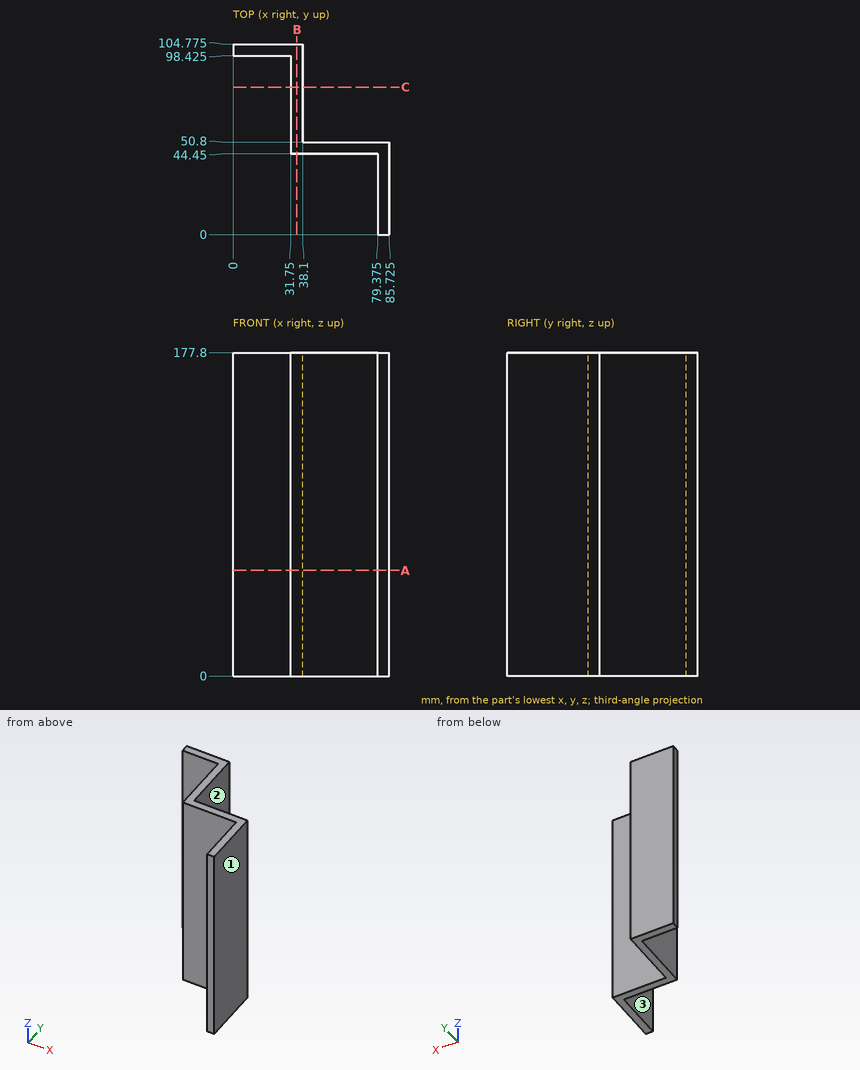
The figure shows three views and two pictorial views of one solid part (mm, origin at its lowest corner). Answer the questions. A direction names the side the tool comes from. Coordinates: 2 decimals unless noted, no trailing zeros. Write each loop counter-clockwise with the first axis right and the second up, starting at its lowest first coordinate (ties: lowest second). Pieces come first, ordered by that corner, then holes. Notation, with made-up numbers: (17, -30) -> (51, -30) arc R29 ccw to (51, 2) -> close; hole circle Ø11 at (-10.5, 24.25). An arc over 180 degrees is marked (long way). Return JSON: item names as keys, results as strings.
(1) The part is cut by section C-C on y = 81. Give the vertices of the cut face in (x, z).
Answers below:
{"outline": "(31.75, 0) -> (38.1, 0) -> (38.1, 177.8) -> (31.75, 177.8) -> close"}
(2) Which of the six approach directions +Z, -Z, +X, -X, +Y, -Y give full straight-line access (tool end or side, diameter ignored) to the marked faces 1, 2 and 3?
Answers below:
{"face 1": "+Z, -Z, +X, +Y, -Y", "face 2": "+Z, -Z, +X, +Y", "face 3": "+Z, -Z, -X, -Y"}
(3) Each of these flat-tipped pins is pushed along its axis until it touches: P1, Ø14.5, axis at x = 61, z = 105.5, coming from the +Y side; P2, Ø6, axis at x = 24.5, z = 120.5, coming from the -Y side (3 decimals); P3, Ø6, axis at x = 41.5, z = 58, coming from the -Y side; P4, Ø6, axis at x = 47, y = 55, coming from the +Z side. Where does it stop, or does it pass through?
Answers below:
{"P1": "y = 50.8", "P2": "y = 98.425", "P3": "y = 44.45", "P4": "through"}
(4) The part is cut by section B-B on x = 35. Give the vertices of the cut face in (y, z) (3 decimals).
Answers below:
{"outline": "(44.45, 0) -> (104.775, 0) -> (104.775, 177.8) -> (44.45, 177.8) -> close"}
(5) Consider line 1 along X through (y, z) = (35, 126.5) (3 decimals); line 2 along X through (y, z) = (51, 11); line 3 along Y through (x, z) = (70, 55.5). Determine where each line is inside the solid, lowest interval first. Write a range as from..to.
Answers below:
{"line 1": "79.375..85.725", "line 2": "31.75..38.1", "line 3": "44.45..50.8"}
(6) The part is cut by section A-A on z = 58. Give the vertices of the cut face in (x, y) (3 decimals).
Answers below:
{"outline": "(0, 98.425) -> (31.75, 98.425) -> (31.75, 44.45) -> (79.375, 44.45) -> (79.375, 0) -> (85.725, 0) -> (85.725, 50.8) -> (38.1, 50.8) -> (38.1, 104.775) -> (0, 104.775) -> close"}
